Model file for the job. Use its own axes, mm. Face numbers are marked on the shaded views. A direction names the side the tool comes from. Round coordinates to 2 decimals unless told otherwise and drop trailing zeros. Loops run counter-clockwise (first coordinate to the right, second up) from the corner with the lowest first, then second, coordinate; pieces in that order, holes last. Notation, with made-up numbers: (-30, 50.25) -> (16, 50.25) arc R18 ccw to (16, 66.25) -> close; hole circle Ø9 at (80.25, 63). An arc over 180 degrees is marked (long way). Use a Markdown table: item, result. Add a question column.
Autodesk Fusion 360 part; units mm, degrees
sketch "Base_Sketch" plane through (0, 0, 0) normal (0, 0, 1) x (1, 0, 0)
  line L0 (33, -21) -> (-33, -21)
  line L1 (-33, -21) -> (-33, 21)
  line L2 (-33, 21) -> (33, 21)
  line L3 (33, 21) -> (33, -21)
  line L4 (33, -21) -> (-33, 21) construction
  line L5 (-33, -21) -> (33, 21) construction
  dimension "d1" = 66
  dimension "d2" = 42
extrude "Extrude1" add sketch "Base_Sketch" along normal blind 12
chamfer "Chamfer1" distance 12 angle 45 2 edges at (33, -21, 6) (33, 21, 6)
sketch "Front_Base_Sketch" plane through (0, 0, 12) normal (0, 0, 1) x (-1, 0, 0)
  line L0 (-33, -9) -> (-21, -21)
  line L1 (-21, -21) -> (33, -21)
  line L2 (33, -21) -> (33, 21)
  line L3 (33, 21) -> (-21, 21)
  line L4 (-21, 21) -> (-33, 9)
  line L5 (-33, 9) -> (-33, -9)
  line L6 (33, -21) -> (21, -21)
  line L7 (21, -21) -> (21, 21)
  line L8 (21, 21) -> (33, 21)
  line L9 (33, 21) -> (33, -21)
  dimension "d6" = 12
extrude "Extrude2" add sketch "Front_Base_Sketch" along normal blind 48 contours L1 L2 L3 L6 L7 L8 L9
fillet "Fillet1" radius 21 2 edges at (-27, -21, 60) (-27, 21, 60)
sketch "Triangle_Sketch" plane through (0, 0, 0) normal (0, 1, 0) x (1, 0, 0)
  line L0 (-21, -54.0075) -> (-21, -12.0075)
  line L1 (-21, -12.0075) -> (33, -12.0075)
  line L2 (33, -12.0075) -> (-21, -54.0075)
  dimension "d10" = 42
  dimension "d11" = 54
extrude "Extrude3" add sketch "Triangle_Sketch" along normal mid plane 12
equation "d11 = 66 mm - 12 mm"
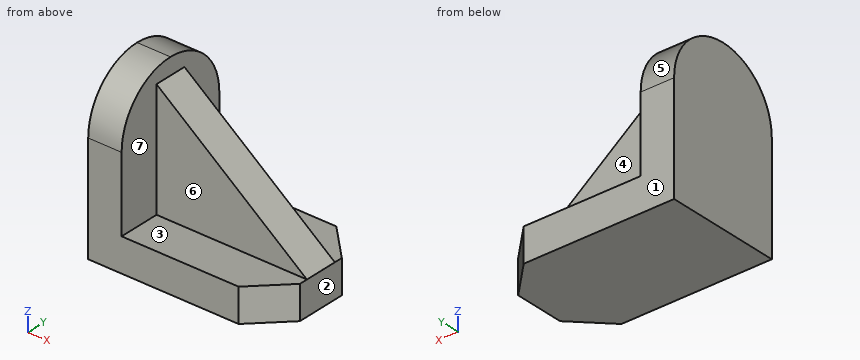
1) Pull direction Y, two halves, no side cores. Call the marked faces 1, 2 and 3: +Y half, -Y half, draft (parallel to the pull), parting line (faces both ways), or undercut.
2) Cut at A-A on x = 3.5. Write the cut outline in (y, z).
3) Tool access for the marked faces 4, 5, 6 and 7: list every direction of +Z, -Z, +X, -X, +Y, -Y with a clear straight run to the whole face (end or side of a thin tool).
4) Pin check, flat tips, straight feed: pin 1 Ø10 at (x, z) = (7, 19) entering from -Y; pin 2 Ø12.5 at (x, y) = (2.5, -0.5) entering from +Z; pin 3 Ø4 at (y, z) = (15, 17.5) entering from +X. Stop position of each tip, or through.
5) Cut at B-B on z = 30. Write the cut outline in (x, y).
6) Wall check: probe 1 along Y at (x, z) = (-14, 47); probe 2 along Z at (x, y) = (23.5, -18); probe 3 along X at (y, z) = (6.5, 29.5). Give the ranges that are in metal, low to high. Write a range as from..to.
Established:
| question | item | result |
|---|---|---|
| 1 | face 1 | +Y half |
| 1 | face 2 | draft |
| 1 | face 3 | undercut |
| 2 | outline | (-21, 0) -> (21, 0) -> (21, 12) -> (-21, 12) -> close; (-6, 12.01) -> (6, 12.01) -> (6, 34.95) -> (-6, 34.95) -> close |
| 3 | face 4 | +Z, +X, +Y |
| 3 | face 5 | +Z, +X, -X, +Y |
| 3 | face 6 | +Z, +X, -Y |
| 3 | face 7 | +Z, +X |
| 4 | pin 1 | stops at y = -6 |
| 4 | pin 2 | stops at z = 40.59 |
| 4 | pin 3 | stops at x = -21 |
| 5 | outline | (-33, -21) -> (-21, -21) -> (-21, -6) -> (9.87, -6) -> (9.87, 6) -> (-21, 6) -> (-21, 21) -> (-33, 21) -> close |
| 6 | probe 1 | y = -6..6 |
| 6 | probe 2 | z = 0..12 |
| 6 | probe 3 | x = -33..-21 |
